Autodesk Inventor part; units mm, degrees
ref_plane "YZ Plane" through (0, 0, 0) normal (1, 0, 0) x (0, 1, 0)
ref_plane "XZ Plane" through (0, 0, 0) normal (0, 1, 0) x (-1, 0, 0)
ref_plane "XY Plane" through (0, 0, 0) normal (0, 0, 1) x (1, 0, 0)
sketch "Sketch1" plane through (0, 0, 0) normal (0, 1, 0) x (-1, 0, 0)
  line L0 (-57.15, -86.36) -> (57.15, -86.36)
  line L1 (57.15, -86.36) -> (57.15, 86.36)
  line L2 (57.15, 86.36) -> (-57.15, 86.36)
  line L3 (-57.15, 86.36) -> (-57.15, -86.36)
  line L4 (-57.15, -86.36) -> (57.15, 86.36) construction
  line L5 (57.15, -86.36) -> (-57.15, 86.36) construction
  point P0 (0, 0)
  dimension "d0" = 114.3
  dimension "d1" = 172.72
extrude "Extrusion1" add sketch "Sketch1" along normal blind 38.1
sketch "Sketch2" plane through (57.15, 0, 86.36) normal (1, 0, 0) x (0, 0, -1)
  line L0 (6.35, 31.75) -> (166.37, 31.75)
  line L1 (166.37, 31.75) -> (166.37, 0)
  line L2 (166.37, 0) -> (6.35, 0)
  line L3 (6.35, 0) -> (6.35, 31.75)
  line L4 (0, 0) -> (172.72, 0)
  line L5 (172.72, 0) -> (172.72, 38.1)
  point P0 (86.36, 0)
  dimension "d4" = 160.02
  dimension "d5" = 31.75
  dimension "d6" = 0
  dimension "d7" = 6.35
extrude "Extrusion2" cut sketch "Sketch2" against normal blind 127
fillet "Fillet1" radius 2.54 4 edges at (0, 38.1, 86.36) (0, 38.1, -86.36) (57.15, 38.1, 0) (-57.15, 38.1, 0)
sketch "Sketch3" plane through (-57.15, 0, 86.36) normal (0, 0, 1) x (1, 0, 0)
  point P0 (57.15, 0)
properties part number "NavX_Box"
Verification items for the finished model (mm, model axes). A direction names the side the tool comes from. Give positions to 0.01 mm unless a question says otherwise; leave off trailing zeros. Order: outer loops, then holes, each group sorted by start corner. A loop starts at its lowest first (then second) coordinate and runs counter-clockwise, first axis right, second up. Notation, with made-up numbers: M 62,-5.75 L 91,-5.75 A19 ccw 91,16.25 Z; hole C 31.5,14.5 d10. An arc over 180 degrees is marked long. Answer in a Markdown table with one row per item. Add a question column.
Item 1: Scan lines: probe 1 along Z at (x, y) = (-51, 15.5); probe 2 along Y at (x, z) = (-12, -77); probe 3 along Z at (x, y) = (9, 36). Record each from-to range of solid material in increasing order. Write a range as from..to.
Item 2: Mould release check, pull along Z, two halves, no side actions. Record for faces 3 (the flat face through (-1, 18, 86.36)), 4 (the flat face through (1, 31.75, 1)), 5 (the flat face through (1, 0, 83)): released by +Z, released by -Z, zero draft, split by the parting line, or undercut.
Item 3: Section check B-B, the plane x = -36. Enter the section's corners in (y, z), and give its area (3 significant figures).
Item 4: Gauge pin test, flat end, axial feed: pin 1 (12 mm diameter, centred on x = 6.5, z = 49.5, fed in from -Y). Record the tip position at first contact, or that the pin passes through.
Item 5: Section check C-C, the plane z = 30. Enter the section's corners in (x, y).
Item 6: Tool access check on faces 1 (the flat face through (57.15, 34, 0)), 2 (the flat face through (1, 16, -80.01)). Record the directions out of +Z, -Z, +X, -X, +Y, -Y that give a thin tool (end or side, any length) a straight path to the whole face; none if there is none.
Item 7: Section check A-A, the plane y = 13. Enter the section's corners in (x, z).
Filled sheet:
| question | item | result |
|---|---|---|
| 1 | probe 1 | z = -86.36..-80.01, 80.01..86.36 |
| 1 | probe 2 | y = 31.75..38.1 |
| 1 | probe 3 | z = -86.32..86.32 |
| 2 | face 3 | released by +Z |
| 2 | face 4 | undercut |
| 2 | face 5 | zero draft |
| 3 | outline | M 0,-86.36 L 35.56,-86.36 A2.54 ccw 38.1,-83.82 L 38.1,83.82 A2.54 ccw 35.56,86.36 L 0,86.36 L 0,80.01 L 31.75,80.01 L 31.75,-80.01 L 0,-80.01 Z |
| 3 | area | 1,500 mm^2 |
| 4 | pin 1 | stops at y = 31.75 |
| 5 | outline | M -57.15,31.75 L 57.15,31.75 L 57.15,35.56 A2.54 ccw 54.61,38.1 L -54.61,38.1 A2.54 ccw -57.15,35.56 Z |
| 6 | face 1 | +Z, -Z, +X, +Y, -Y |
| 6 | face 2 | +X, -X, -Y |
| 7 | outline | M -57.15,-86.36 L 57.15,-86.36 L 57.15,-80.01 L -57.15,-80.01 Z; M -57.15,80.01 L 57.15,80.01 L 57.15,86.36 L -57.15,86.36 Z |
